```python
from build123d import *

# Parameters (mm, degrees)
F0_W      = 78
F0_H      = 43
F1_DEPTH  = 21
F2_R      = 1.35
F3_DEPTH  = 19
F5_DEPTH  = 19
F7_R      = 3.2
F7_R_2    = 1.5
F7_R_3    = 2.625
F8_DEPTH  = 10
F9_W      = 112
F9_H      = 21
F10_DEPTH = 6
F11_R     = 3.3
F12_DEPTH = 49.001
F13_R     = 3
F14_W     = 15
F14_H     = 12
F15_DEPTH = 3
F16_W     = 74
F16_H     = 11
F17_DEPTH = 7
F19_R     = 3.75
F20_DEPTH = 7
F22_W     = 8.5
F22_H     = 8
F23_DEPTH = 3.5


with BuildPart() as f1:
    # F0 (on Top) → F1 (new body)
    with BuildSketch(Plane.XY):
        Rectangle(F0_W, F0_H)
    extrude(amount=F1_DEPTH)

    # F2 (on face) → F3 (cut)
    with BuildSketch(Plane.XY.offset(21)):
        with BuildLine():
            Line((31, 17.5), (-31, 17.5))
            Line((-31, 17.5), (-31, -17.5))
            Line((-31, -17.5), (31, -17.5))
            ThreePointArc((31, -17.5), (32.1715728753, -14.6715728753), (35, -13.5))
            Line((35, -13.5), (35, 13.5))
            ThreePointArc((35, 13.5), (32.1715728753, 14.6715728753), (31, 17.5))
        make_face()
        with Locations((-35, 17.5)):
            Circle(F2_R)
        with Locations((35, 17.5)):
            Circle(F2_R)
        with Locations((-35, -17.5)):
            Circle(F2_R)
        with Locations((35, -17.5)):
            Circle(F2_R)
    extrude(amount=-F3_DEPTH, mode=Mode.SUBTRACT)

    # F4 (on face) → F5 (cut)
    with BuildSketch(Plane.XY.offset(21)):
        with BuildLine():
            ThreePointArc((-32.65, 17.5), (-33.5256357302, 15.6700409841), (-35.5, 15.2038074994))
            Line((-35.5, 15.2038074994), (-35.5, -15.2038074994))
            ThreePointArc((-35.5, -15.2038074994), (-33.5256357302, -15.6700409841), (-32.65, -17.5))
            Line((-32.65, -17.5), (-31, -17.5))
            Line((-31, -17.5), (-31, 17.5))
            Line((-31, 17.5), (-32.65, 17.5))
        make_face()
    extrude(amount=-F5_DEPTH, mode=Mode.SUBTRACT)

    # F7 (on face) → F8 (cut)
    with BuildSketch(Plane.YZ.offset(39)):
        with Locations((4, 6)):
            Circle(F7_R)
        with Locations((14.5, 6)):
            Circle(F7_R_2)
        with Locations((-11, 6)):
            Circle(F7_R_3)
    extrude(amount=-F8_DEPTH, mode=Mode.SUBTRACT)

    # F9 (on face) → F10 (join)
    with BuildSketch(Plane(origin=(0, 21.5, 0), x_dir=(-1, 0, 0), z_dir=(0, 1, 0))):
        with Locations((0, 10.5)):
            Rectangle(F9_W, F9_H)
    extrude(amount=F10_DEPTH)

    # F11 (on face) → F12 (cut, through all)
    with BuildSketch(Plane(origin=(0, 27.5, 0), x_dir=(-1, 0, 0), z_dir=(0, 1, 0))):
        with Locations((50.75, 10.5)):
            Circle(F11_R)
        with Locations((-50.75, 10.5)):
            Circle(F11_R)
    extrude(amount=-F12_DEPTH, mode=Mode.SUBTRACT)

    # F13
    f13_edges = [f1.edges().sort_by_distance(p)[0] for p in [
        (56, 24.5, 21),
        (56, 24.5, 0),
        (-56, 24.5, 0),
        (-56, 24.5, 21),
    ]]
    fillet(f13_edges, radius=F13_R)

    # F14 (on face) → F15 (cut)
    with BuildSketch(Plane(origin=(35, 0, 0), x_dir=(0, -1, 0), z_dir=(-1, 0, 0))):
        with Locations((-4, 8)):
            Rectangle(F14_W, F14_H)
    extrude(amount=-F15_DEPTH, mode=Mode.SUBTRACT)

    # F16 (on face) → F17 (cut)
    with BuildSketch(Plane(origin=(0, 27.5, 0), x_dir=(-1, 0, 0), z_dir=(0, 1, 0))):
        with Locations((0, 10.5)):
            Rectangle(F16_W, F16_H)
    extrude(amount=-F17_DEPTH, mode=Mode.SUBTRACT)

    # F19 (on offset) → F20 (cut)
    with BuildSketch(Plane(origin=(30, 0, 0), x_dir=(0, -1, 0), z_dir=(-1, 0, 0))):
        with Locations((11, 6)):
            Circle(F19_R)
    extrude(amount=-F20_DEPTH, mode=Mode.SUBTRACT)

    # F22 (on face) → F23 (cut, through all)
    with BuildSketch(Plane(origin=(-39, 0, 0), x_dir=(0, -1, 0), z_dir=(-1, 0, 0))):
        with Locations((2.3, 11)):
            Rectangle(F22_W, F22_H)
    extrude(amount=-F23_DEPTH, mode=Mode.SUBTRACT)


solid = f1.part
```
Could you check a few things on this model? Use its own coordinates, in mm. A direction names the side the tool comes from. Coordinates: 2 decimals unless noted, no trailing zeros. Order: outer loops, then holes, each group sorted by start corner. A loop starts at its lowest first (then second) coordinate and runs counter-clockwise, first axis right, second up. Notation, with made-up numbers: M 84,-9 L 88,-9 A13 ccw 88,9 Z; hole C -16.5,-19.5 d11. An arc over 180 degrees is marked long. Use a Markdown table: item, result. Add a question column.
Q1. We'd pull the mould along Z, two halves only. Please class faces 5 (the flat face through (35, -17, 2)), 6 (the cylindrical face through (55.14, 24.54, 0.9)), 7 (the flat face through (-37, -2, 15)): pulls with the +Z half, pulls with the -Z half, needs draft (parallel to the pull), parting line crosses it, or undercut.
Q2. I want a section at B-B on x = -50.75. List the corners of the cut face in (y, z) for me, then the cut area to 3 significant figures.
Q3. I want a section at C-C on y = 23.5. List the corners of the cut face in (x, z) for me, then the cut area to 3 significant figures.
Q4. I want a section at D-D on x = -14. List the corners of the cut face in (y, z) for me, then the cut area to 3 significant figures.
Q5. I want a section at A-A on y = -11. List the corners of the cut face in (x, z) for me (3 decimals).
Q6. I'm going to push flat-ended pins straight in: pin 1 (1.5 mm diameter, centred on y = 2.5, z = 16, fed in from +X); pin 2 (9.5 mm diameter, centred on y = -3, z = 14, fed in from -X); pin 3 (0.8 mm diameter, centred on x = -35.5, y = -17, fed in from +Z). Where does each tip first touch, or does it pass through?
Q7. Which directions (+Z, -Z, +X, -X, +Y, -Y) give clear straight access to the entire face, cutting with the end or side of a thin tool? Please do faces 1 (the flat face through (-37, 1.95, 11)), 2 (the cylindrical face through (35.603, -14.577, 7.126)), 3 (the flat face through (-39, 4, 10)), 4 (the flat face through (37, 24, 10)).
Q8. If I drill on L1, parallel to Y at x = -35, z = 9.75; L2, parallel to Y at x = 35.2, z = 6; L3, parallel to Y at x = -11.5, z = 12.25, over which ranges is the centre line in solid material (lowest first)?
Checked values:
| question | item | result |
|---|---|---|
| 1 | face 5 | pulls with the +Z half |
| 1 | face 6 | pulls with the -Z half |
| 1 | face 7 | undercut |
| 2 | outline | M 21.5,0 L 27.5,0 L 27.5,7.2 L 21.5,7.2 Z; M 21.5,13.8 L 27.5,13.8 L 27.5,21 L 21.5,21 Z |
| 2 | area | 86.4 mm² |
| 3 | outline | M -56,3 A3 ccw -53,0 L 53,0 A3 ccw 56,3 L 56,18 A3 ccw 53,21 L -53,21 A3 ccw -56,18 Z; hole C -50.75,10.5 d6.6; hole M -37,5 L 37,5 L 37,16 L -37,16 Z; hole C 50.75,10.5 d6.6 |
| 3 | area | 1,460 mm² |
| 4 | outline | M -21.5,0 L 27.5,0 L 27.5,5 L 20.5,5 L 20.5,16 L 27.5,16 L 27.5,21 L 17.5,21 L 17.5,2 L -17.5,2 L -17.5,21 L -21.5,21 Z |
| 4 | area | 287 mm² |
| 5 | outline | M -39,0 L 39,0 L 39,3.375 L 37,3.375 L 37,2.25 L 35,2.25 L 35,2 L -35.5,2 L -35.5,21 L -39,21 Z; M 35,9.75 L 37,9.75 L 37,8.625 L 39,8.625 L 39,21 L 35,21 Z |
| 6 | pin 1 | x = 39 |
| 6 | pin 2 | x = -39 |
| 6 | pin 3 | z = 2 |
| 7 | face 1 | -X |
| 7 | face 2 | none |
| 7 | face 3 | +Z, -Z, -X, -Y |
| 7 | face 4 | +Y |
| 8 | L1 | -21.5 to -18.85, -16.15 to -15.15, 15.15 to 16.15, 18.85 to 20.5 |
| 8 | L2 | -21.5 to -18.84, -16.16 to -14.75, -7.25 to -3.5, 11.5 to 13, 16 to 16.16, 18.84 to 20.5 |
| 8 | L3 | -21.5 to -17.5, 17.5 to 20.5 |
